from build123d import *

# Parameters (mm, degrees)
CHAFL_N2_SIZE         = 0.3
CHAFL_N2_SIZE2        = 0.212132034
CHAFL_N3_SIZE         = 0.3
CORTAR_EXTRUIR2_DEPTH = 1


with BuildPart() as part:
    # Croquis1 → Revolución1 (revolve)
    with BuildSketch(Plane.XY, mode=Mode.PRIVATE) as revoluci_n1_sk:
        Polygon((0, 0), (3.2, 0), (1.5, -1.7), (1.5, -6), (0, -6), align=None)
    revolve(revoluci_n1_sk.sketch.rotate(Axis((0, 0, 0), (0, -1, 0)), 90), axis=Axis((0, 0, 0), (0, -1, 0)))

    # Chaflán2
    chafl_n2_edges = [part.edges().sort_by_distance(p)[0] for p in [
        (0, 0, -3.2),
    ]]
    chafl_n2_side = [part.faces().sort_by_distance(p)[0] for p in [
        (0, -0.85, -2.35),
    ]]
    chamfer(chafl_n2_edges, length=CHAFL_N2_SIZE, length2=CHAFL_N2_SIZE2, reference=chafl_n2_side[0])

    # Chaflán3
    chafl_n3_edges = [part.edges().sort_by_distance(p)[0] for p in [
        (0, -6, -1.5),
    ]]
    chamfer(chafl_n3_edges, length=CHAFL_N3_SIZE)

    # Croquis3 → Cortar-Extruir2 (cut)
    with BuildSketch(Plane(origin=(0, 0, 0), x_dir=(1, 0, 0), z_dir=(0, 1, 0))):
        Polygon((-0.721687836, 1.25), (-1.443375673, 0), (-0.721687836, -1.25), (0.721687836, -1.25), (1.443375673, 0), (0.721687836, 1.25), align=None)
    extrude(amount=-CORTAR_EXTRUIR2_DEPTH, mode=Mode.SUBTRACT)


solid = part.part
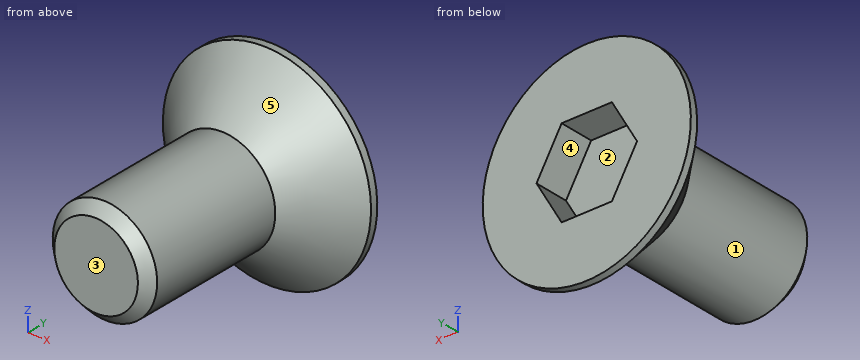
Check sheet for the modelled part. Datum: model origin and axes. Units: mm. Face numbers are marked on the shaded views. A direction names the side the tool comes from. Give positions to 0.01 mm unless a question says otherwise; leave off trailing zeros. Write each loop counter-clockwise with the first axis right and the second up, starting at its lowest first coordinate (ties: lowest second). Pieces come first, ordered by that corner, then holes. Notation, with made-up numbers: (84.25, 30) -> (133.25, 30) arc R22 cw to (133.25, 59) -> close; hole circle Ø2 at (16, 12.5). An arc over 180 degrees is marked (long way). Use one line per item in the form item = value. Start each with the question number.
1. Section check B-B (y = -4.6). Record the cut outline in (x, z).
2. Mould release check, pull along Z, two halves, no side actions. Record for the marked faces 1, 2 and 3: pulls with the +Z half, pulls with the -Z half, needs draft (parallel to the pull), parting line crosses it, or undercut.
3. Access from +Z, -Z, +X, -X, +Y, -Y to the whole of each face (thin tool, end or side, straight path). Record for the marked faces 4 and 5.
4. Thickness scan on line 1 along X through (y, z) = (-4.55, 0.05); line 2 along Z through (x, y) = (0.35, -4.35); line 3 along Y through (x, z) = (0.5, 0). Record the ranges inside material, lowest first. Write a range as from..to.
5. Section check A-A (y = -0.5). Record the cut outline in (x, z).
6. Go/stop test with flat-tipped pins: P1, Ø1, axis at x = -0.5, y = -2, coming from the +Z side; P2, Ø1.5, axis at x = -2.5, z = -1.5, coming from the -Y side. Record where each tip stops, or that it passes through.
Conclusion:
q1.outline = circle Ø3 at (0, 0)
q2.face_1 = parting line crosses it
q2.face_2 = undercut
q2.face_3 = needs draft
q3.face_4 = +Y
q3.face_5 = -Y
q4.line_1 = -1.5..1.5
q4.line_2 = -1.46..1.46
q4.line_3 = -6..-1
q5.outline = circle Ø5.4 at (0, 0); hole (-1.44, 0) -> (-0.72, -1.25) -> (0.72, -1.25) -> (1.44, 0) -> (0.72, 1.25) -> (-0.72, 1.25) -> close
q6.P1 = 1.64
q6.P2 = -1.03
